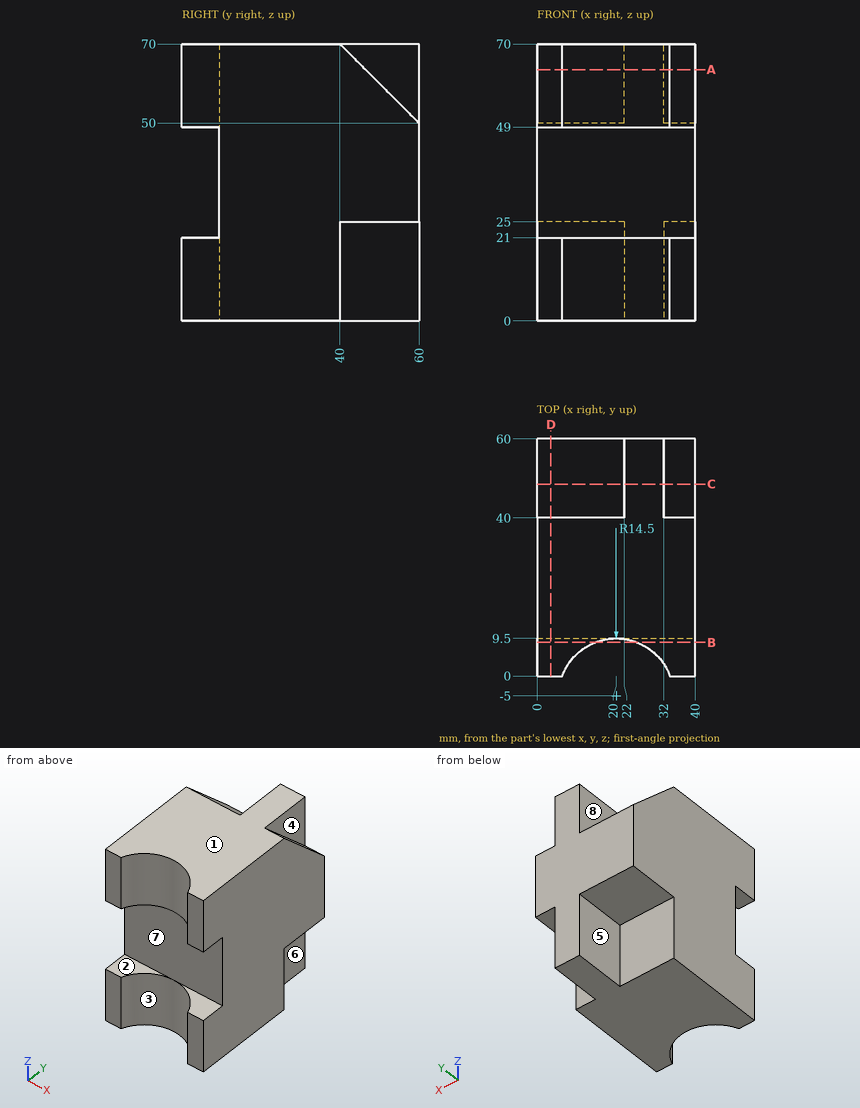
Study the drawing (mm; zero at the part's minimum x, y, z) and answer. A direction names the side the tool comes from. Coordinates: 2 decimals unless noted, no trailing zeros. Write each loop counter-clockwise with the first axis right and the second up, starting at its lowest first coordinate (ties: lowest second). Pieces come first, ordered by that corner, then holes. Notation, with made-up numbers: M 54,-40 L 66,-40 A23 cw 66,-7 Z; hole C 0,-32 d5. An arc over 180 degrees is marked long. Use a Markdown table: item, result. Add a question column.
1. Given P1, Ø10, axis at x = 23.5, z = 10.5, coming from the -Y side; P2, Ø2.5, axis at x = 36.5, y = 48.5, coming from the -Z side; P3, Ø1, axis at x = 5, z = 55.5, coming from the +Y side, each flat-ended and moving along its own axis, determine where each tip first touches the part or whether it passes through.
2. Straight lines are drawn through the part: line 1 along Z through (x, y) = (36.5, 6); line 2 along X through (y, z) = (45.5, 21); line 3 along Y through (x, z) = (19, 30). For each, find the intervals that lie inside material, in ascending order. Write a range as [from, to].
3. Section C-C (y = 48.5) is taken. Give the vertices of the cut face in (x, z), plus the area to 4 significant figures.
4. Section D-D (x = 3.5) is taken. Give the vertices of the cut face in (y, z).
5. Section B-B (y = 8.5) is taken. Give the vertices of the cut face in (x, z), plus the area to 3 significant figures.
6. Which of the six approach directions +Z, -Z, +X, -X, +Y, -Y give full straight-line access (tool end or side, diameter ignored) to the marked faces 4, 5, 6, 7 and 8?
7. For a pull along Z with two mould halves and no side action, classify the marked faces 1, 2 and 3 as +Z half, -Z half, draft (parallel to the pull), parting line (faces both ways), or undercut.
8. Section A-A (z = 63.5) is taken. Give the vertices of the cut face in (x, y).
Data:
| question | item | result |
|---|---|---|
| 1 | P1 | stops at y = 6.75 |
| 1 | P2 | stops at z = 25 |
| 1 | P3 | stops at y = 55 |
| 2 | line 1 | z = [0, 21], [49, 70] |
| 2 | line 2 | x = [22, 32] |
| 2 | line 3 | y = [9.5, 60] |
| 3 | outline | M 0,25 L 22,25 L 22,0 L 32,0 L 32,25 L 40,25 L 40,61.5 L 32,61.5 L 32,70 L 22,70 L 22,61.5 L 0,61.5 Z |
| 3 | area | 1,795 mm2 |
| 4 | outline | M 0,0 L 40,0 L 40,25 L 60,25 L 60,50 L 40,70 L 0,70 L 0,49 L 9.5,49 L 9.5,21 L 0,21 Z |
| 5 | outline | M 0,0 L 14.71,0 L 14.71,21 L 0,21 Z; M 0,49 L 14.71,49 L 14.71,70 L 0,70 Z; M 25.29,0 L 40,0 L 40,21 L 25.29,21 Z; M 25.29,49 L 40,49 L 40,70 L 25.29,70 Z |
| 5 | area | 1,240 mm2 |
| 6 | face 4 | +Z, +X, +Y |
| 6 | face 5 | -Z, -X, +Y |
| 6 | face 6 | -Z, +X, +Y |
| 6 | face 7 | +X, -X, -Y |
| 6 | face 8 | +Z, -X, +Y |
| 7 | face 1 | +Z half |
| 7 | face 2 | undercut |
| 7 | face 3 | draft |
| 8 | outline | M 0,0 L 6.39,0 A14.5 cw 33.61,0 L 40,0 L 40,46.5 L 32,46.5 L 32,60 L 22,60 L 22,46.5 L 0,46.5 Z |
